```python
from build123d import *

# Parameters (mm, degrees)
F0_W     = 50
F0_H     = 50
F1_DEPTH = 5
F3_DEPTH = 10
F4_DEPTH = 5
F6_DEPTH = 5


with BuildPart() as f1:
    # F0 (on Top) → F1 (new body, symmetric)
    with BuildSketch(Plane.XY):
        Rectangle(F0_W, F0_H)
    extrude(amount=F1_DEPTH, both=True)

    # F2 (on face) → F3 (cut)
    with BuildSketch(Plane.XY.offset(5)):
        Polygon((0.262668, 14.382005), (10.857864, 25), (-25, 25), (-25, -15), (-12.386651, -12.820839), align=None)
        Polygon((25, -25), (25, 10.857864), (14.739396, -17.332914), (-5, -25), align=None)
        Polygon((25, 25), (10.857864, 25), (25, 10.857864), align=None)
    extrude(amount=-F3_DEPTH, mode=Mode.SUBTRACT)

    # F1_face (on face) → F4 (cut)
    with BuildSketch(Plane.XY.offset(5)):
        Polygon((-25, -15), (-25, -25), (-5, -25), (14.739396, -17.332914), (25, 10.857864), (10.857864, 25), (0.262668, 14.382005), (-12.386651, -12.820839), align=None)
    extrude(amount=-F4_DEPTH, mode=Mode.SUBTRACT)

    # F5 (on face) → F6 (join)
    with BuildSketch(Plane.XY):
        Polygon((-11.219984, -13.763648), (-10.886651, -12.820839), (-12.386651, -12.820839), align=None)
        Polygon((1.762668, 14.382005), (0.262668, 14.382005), (-12.386651, -12.820839), (-10.886651, -12.820839), align=None)
        Polygon((-11.219984, -13.763648), (-12.386651, -12.820839), (-25, -15), (-25, -16.14437), align=None)
        Polygon((-5, -25), (-5.283205, -23.5), (-25, -23.5), (-25, -25), align=None)
        Polygon((14.739396, -17.332914), (13.951547, -16.028926), (-5.283205, -23.5), (-5, -25), align=None)
        Polygon((24.593647, 9.741419), (23.668068, 10.666997), (13.951547, -16.028926), (14.739396, -17.332914), align=None)
        Polygon((10.857864, 25), (10.097283, 24.237782), (10.857864, 23.477201), (23.668068, 10.666997), (24.593647, 9.741419), (25, 10.857864), align=None)
    extrude(amount=F6_DEPTH)


solid = f1.part
```
Verification items for the finished model (mm, model axes). A direction names the side the tool comes from. Give positions to 0.01 mm unless a question says otherwise; leave off trailing zeros. Loops run counter-clockwise (first coordinate to the right, second up) from the corner with the lowest first, then second, coordinate; pieces in that order, holes last. Notation, with made-up numbers: M 58.5,77 L 99.5,77 A32 ccw 99.5,110 Z; hole C 84,33.25 d10. An arc over 180 degrees is marked long. One line per question, with ' | ' between items.
Item 1: Section check C-C, the plane y = -5. Record the cut outline in (x, z), plus the area to 3 significant figures.
Completed:
outline: M -8.75,-5 L 19.23,-5 L 19.23,5 L 17.97,5 L 17.97,0 L -7.25,0 L -7.25,5 L -8.75,5 Z | area: 154 mm^2
Item 2: Thickness scan on line 1 (X direction, y = 2, z = 4.75); line 2 (Z direction, x = 1.5, y = 12); line 3 (X direction, y = -7, z = 3.5). Record the ranges inside material, lowest first. Write a range as [from, to].
Completed:
line 1: x = [-5.49, -3.99], [20.51, 21.78] | line 2: z = [-5, 0] | line 3: x = [-9.68, -8.18], [17.24, 18.5]
Item 3: Section check B-B, the plane z = -2.5. Record the cut outline in (x, y), plus the area to 3 significant figures.
Completed:
outline: M -25,-25 L -5,-25 L 14.74,-17.33 L 25,10.86 L 10.86,25 L 0.26,14.38 L -12.39,-12.82 L -25,-15 Z | area: 1,250 mm^2
Item 4: Draft check along X on faces 1 (the face through (16.788, 17.547, 2.465)), 2 (the face through (-7.7, -3.1, 5)), 3 (the face through (-18.605, -13.895, -0.07)). Enter one of: +X half, -X half, draft (parallel to the pull), parting line (faces both ways), or undercut.
Completed:
face 1: undercut | face 2: draft | face 3: -X half
Item 5: Section check D-D, the plane x = 9.5. Record the cut outline in (y, z).
Completed:
outline: M -19.37,-5 L 23.64,-5 L 23.64,0 L -17.76,0 L -17.76,5 L -19.37,5 Z
Item 6: Depth check by flat-ended pin: P1, Ø2, axis at y = 6.5, z = -1.5, coming from the +X side; P2, Ø6, axis at x = 18.5, z = -3, coming from the +Y side; P3, Ø6, axis at x = 8.5, z = 1, coming from the -Y side. Enter the tip coordinate at first touch or a pass-through.
Completed:
P1: stops at x = 23.78 | P2: stops at y = 20.36 | P3: stops at y = -20.92
Item 7: Tool access check on faces 4 (the face through (-25, -20, -1)), 5 (the face through (1, 14.382, 2)), 6 (the face through (-18.21, -14.97, 2.46)), 7 (the face through (-15, -25, 0)), 8 (the face through (-15, -23.5, 2)). Record the directions out of +Z, -Z, +X, -X, +Y, -Y that give a thin tool (end or side, any length) a straight path to the whole face; none if there is none.
Completed:
face 4: +Z, -Z, -X, +Y, -Y | face 5: +Z, -X, +Y | face 6: +Z | face 7: +Z, -Z, +X, -X, -Y | face 8: +Z, -X
Item 8: Section check A-A, the plane z = 1.5. Record the cut outline in (x, y), plus the area to 3 significant figures.
Completed:
outline: M -25,-25 L -5,-25 L 14.74,-17.33 L 24.59,9.74 L 25,10.86 L 10.86,25 L 10.1,24.24 L 23.67,10.67 L 13.95,-16.03 L -5.28,-23.5 L -25,-23.5 Z; M -25,-16.14 L -11.22,-13.76 L -10.89,-12.82 L 1.76,14.38 L 0.26,14.38 L -12.39,-12.82 L -25,-15 Z | area: 174 mm^2
